Design review of the part shown in the three views and the two pictorial views. Dimensions are in mm from the part's minimum x, y and z. Round coordinates to 2 decimals unless told otherwise and drop trailing zeros. Write each loop counter-clockwise with the first axis right and the second up, starting at its lowest first coordinate (ties: lowest second). Pieces come first, ordered by that corner, then holes. Notation, with made-up numbers: (8, 72) - (30, 72) arc R23 ccw to (30, 100) - close; hole circle Ø7 at (31.5, -34.5). An arc over 180 degrees is marked (long way). One line per item, written item: value. Start each with the question number.
Q1. Add section A-A on z = 169.5. Write out the cut boundary in (x, y), and give its area (3 significant figures).
Q2. Add section B-B on y = 3. Give the number of separate pieces and of enclosed holes in the cut face, and give its area (3 significant figures).
Q3. For probe 1 along X at (y, z) = (4.25, 260.35); probe 2 along Z at (x, y) = (146.05, 3.75); probe 3 along X at (y, z) = (5, 273.05), list the stretches that pass through material, from the lowest coordinate up.
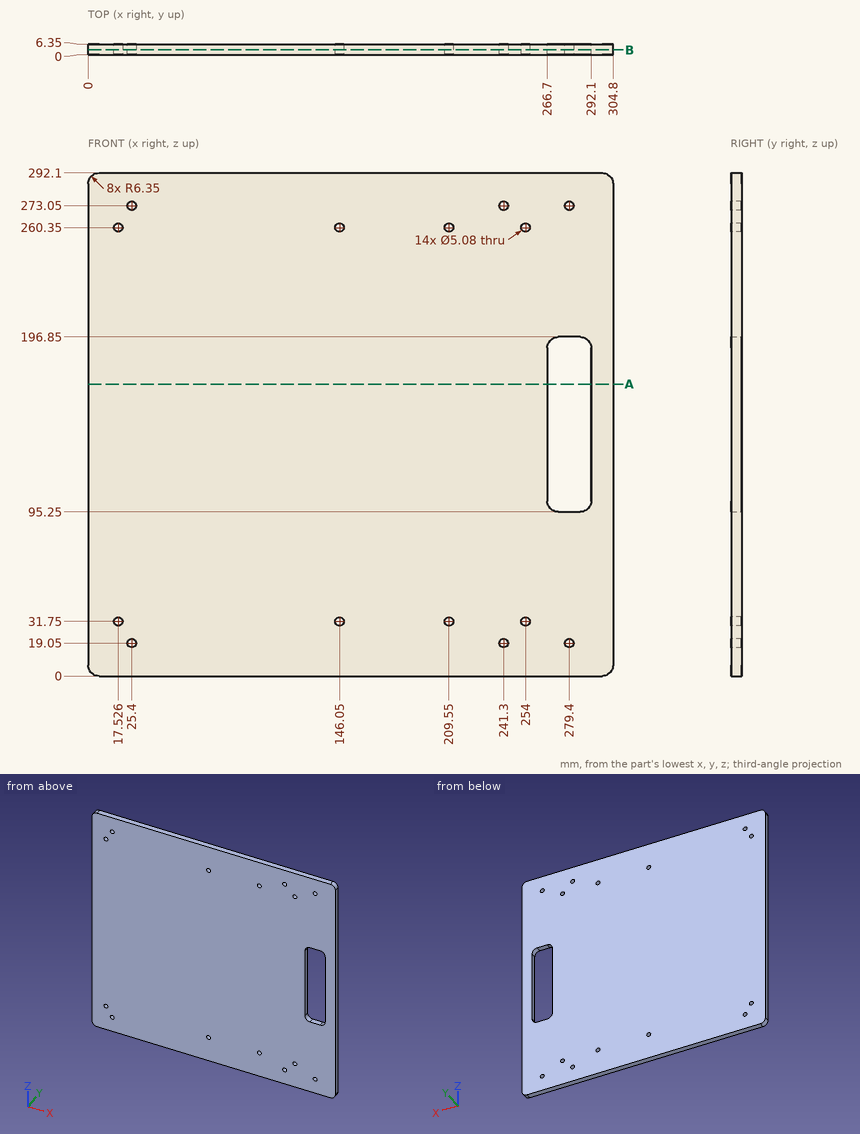
Result set:
1. outline: (0, 0) - (266.7, 0) - (266.7, 6.35) - (0, 6.35) - close; (292.1, 0) - (304.8, 0) - (304.8, 6.35) - (292.1, 6.35) - close
1. area: 1,770 mm^2
2. separate pieces: 1
2. enclosed holes: 15
2. area: 86,200 mm^2
3. probe 1: x = 0 to 14.99, 20.07 to 143.51, 148.59 to 207.01, 212.09 to 251.46, 256.54 to 304.8
3. probe 2: z = 0 to 29.21, 34.29 to 257.81, 262.89 to 292.1
3. probe 3: x = 0 to 22.86, 27.94 to 238.76, 243.84 to 276.86, 281.94 to 304.8
